Autodesk Inventor part; units mm, degrees
ref_plane "YZ Plane" through (0, 0, 0) normal (1, 0, 0) x (0, 1, 0)
ref_plane "XZ Plane" through (0, 0, 0) normal (0, 1, 0) x (-1, 0, 0)
ref_plane "XY Plane" through (0, 0, 0) normal (0, 0, 1) x (1, 0, 0)
sketch "Sketch1" plane through (0, 0, 0) normal (0, 1, 0) x (-1, 0, 0)
  line L0 (0, 0) -> (44.45, 0)
  line L1 (44.45, 0) -> (44.45, -44.45)
  line L2 (44.45, -44.45) -> (0, -44.45)
  line L3 (0, -44.45) -> (0, 0)
  dimension "d0" = 44.45
  dimension "d1" = 44.45
extrude "Extrusion1" add sketch "Sketch1" along normal blind 3.175
sketch "Sketch2" plane through (-44.45, 0, 0) normal (0, 0, 1) x (1, 0, 0)
  line L0 (9.525, 50.8) -> (34.925, 50.8)
  line L1 (44.45, 0) -> (0, 0)
  line L2 (22.225, 50.8) -> (22.225, 54.352)
  line L3 (22.225, 0) -> (22.225, -5.76)
  line L4 (9.525, 50.8) -> (0.0188, 3.175)
  line L5 (0.0188, 3.175) -> (44.4312, 3.175)
  line L6 (44.4312, 3.175) -> (34.925, 50.8)
  line L7 (0, 3.175) -> (44.45, 3.175)
  dimension "d4" = 25.4
  dimension "d5" = 50.8
  dimension "d6" = 0
  dimension "d9" = 0
extrude "Extrusion2" add sketch "Sketch2" against normal blind 3.175
sketch "Sketch3" plane through (0, 0, 0) normal (0, -1, 0) x (1, 0, 0)
  line L0 (-25.273, 0) -> (-25.273, 3.175)
  line L1 (-19.177, 3.175) -> (-19.177, 0)
  line L2 (-19.177, 0) -> (-25.273, 0)
  line L3 (0, 0) -> (-44.45, 0)
  line L4 (-25.273, 3.175) -> (-19.177, 3.175)
  line L5 (0, -44.45) -> (0, 0)
  dimension "d10" = 3.175
  dimension "d13" = 6.096
  dimension "d14" = 19.177
extrude "Extrusion3" add sketch "Sketch3" against normal up to surface (50.8 mm away)
properties part number "Bottom Elevator Bracket"
Can you work these out from the model? Positions are in its coordinate system, mm. A direction names the side the tool comes from. Round coordinates to 2 decimals unless told otherwise and drop trailing zeros. Loops run counter-clockwise (first coordinate to the right, second up) from the corner with the lowest first, then second, coordinate; pieces in that order, holes last. Notation, with made-up numbers: M -9,61 L 1,61 A22 cw 1,89 Z; hole C 64.5,78.25 d6. An arc over 180 degrees is marked long. Answer as a JSON object with one key per item and string values. Group by question number.
Q1. Imagine slicing it at B-B, the plane x = -28. Please give me the cut outline in (y, z) (3 decimals).
Q2. Imagine slicing it at C-C, the plane z = -11. Please give me the cut outline in (x, y) (3 decimals), then the cut area to 3 significant figures.
Q3. Will these pins go through, and if not, where does the flat tip stop? pin 1 (1.5 mm diameter, centred on x = -35, y = 30, fed in from -Z) (3 decimals); pin 2 (1 mm diameter, centred on y = 34, z = 2, fed in from -X); pin 3 (1.5 mm diameter, centred on x = -38.5, y = 31.5, fed in from +Z); pin 4 (2 mm diameter, centred on y = 37, z = -4.5, fed in from -X).
Q4. Imagine slicing it at D-D, the plane y = 20. Please give me the cut outline in (x, z) (3 decimals), then the cut area to 3 significant figures.
Q5. Please list where these lines run through material, in increasing order: L1, parallel to Y at x = -4, z = -13.5 (3 decimals); L2, parallel to Z at x = -39, y = 7 (3 decimals); L3, parallel to X at y = 24, z = 0.5.
Q6. On a 3-axis mill with a long thin cutter (end or side, diameter ignored), from which of +Z, -Z, +X, -X, +Y, -Y can I reach the whole of each face in a straight line? I mean faces 1 (the flat face through (-22, 3.175, -22)), 2 (the flat face through (-33, 19, 0)), 3 (the flat face through (-12, 25, 0)). Say none if no direction works.
Q7. Imagine slicing it at A-A, the plane y = 31.5. Please give me the cut outline in (x, z) (3 decimals).
Findings:
{
 "1": {"outline": "M 0,-44.45 L 3.175,-44.45 L 3.175,-3.175 L 50.8,-3.175 L 50.8,0 L 0,0 Z"},
 "2": {"outline": "M -44.45,0 L 0,0 L 0,3.175 L -44.45,3.175 Z", "area": "141 mm2"},
 "3": {"pin 1": "stops at z = -3.175", "pin 2": "stops at x = -25.27", "pin 3": "stops at z = 0", "pin 4": "passes through"},
 "4": {"outline": "M -41.073,-3.175 L -3.377,-3.175 L -3.377,0 L -19.177,0 L -19.177,3.175 L -25.273,3.175 L -25.273,0 L -41.073,0 Z", "area": "139 mm2"},
 "5": {"L1": "y = 0 to 3.175", "L2": "z = -3.175 to 0", "L3": "x = -25.27 to -19.18"},
 "6": {"face 1": "-Z, +X, -X, +Y", "face 2": "+Z, -X, +Y, -Y", "face 3": "+Z, +X, +Y, -Y"},
 "7": {"outline": "M -38.777,-3.175 L -5.673,-3.175 L -5.673,0 L -19.177,0 L -19.177,3.175 L -25.273,3.175 L -25.273,0 L -38.777,0 Z"}
}
